from build123d import *

# Parameters (mm, degrees)
SKETCH1_W           = 55
SKETCH1_H           = 35
BOSS_EXTRUDE1_DEPTH = 1.5
SKETCH2_W           = 15
SKETCH2_H           = 41
BOSS_EXTRUDE2_DEPTH = 1.5
SKETCH3_R           = 1.125
CUT_EXTRUDE1_DEPTH  = 10


with BuildPart() as part:
    # Sketch1 → Boss-Extrude1 (new body)
    with BuildSketch(Plane(origin=(0, 0, 0), x_dir=(1, 0, 0), z_dir=(0, 1, 0))):
        Rectangle(SKETCH1_W, SKETCH1_H)
    extrude(amount=BOSS_EXTRUDE1_DEPTH)

    # Sketch2 → Boss-Extrude2 (add)
    with BuildSketch(Plane(origin=(0, 0, 0), x_dir=(1, 0, 0), z_dir=(0, 1, 0))):
        with Locations((35, 0)):
            Rectangle(SKETCH2_W, SKETCH2_H)
        with Locations((-35, 0)):
            Rectangle(SKETCH2_W, SKETCH2_H)
    extrude(amount=BOSS_EXTRUDE2_DEPTH)

    # Sketch3 → Cut-Extrude1 (cut)
    with BuildSketch(Plane(origin=(0, 0, 0), x_dir=(1, 0, 0), z_dir=(0, 1, 0))):
        with Locations(Location((-39.5, -16.5, 0), (0, 0, 270))):
            Circle(SKETCH3_R)
        with Locations(Location((-39, -7.5, 0), (0, 0, 270))):
            Circle(SKETCH3_R)
        with Locations(Location((-39, 7.5, 0), (0, 0, 270))):
            Circle(SKETCH3_R)
        with Locations(Location((-39.5, 16.5, 0), (0, 0, 270))):
            Circle(SKETCH3_R)
        with Locations(Location((-18, 15, 0), (0, 0, 270))):
            Circle(SKETCH3_R)
        with Locations(Location((18, 15, 0), (0, 0, 270))):
            Circle(SKETCH3_R)
        with Locations(Location((-18, -15, 0), (0, 0, 270))):
            Circle(SKETCH3_R)
        with Locations(Location((18, -15, 0), (0, 0, 270))):
            Circle(SKETCH3_R)
    cut_extrude1 = extrude(amount=CUT_EXTRUDE1_DEPTH, mode=Mode.SUBTRACT)

    # Mirror1: Cut-Extrude1 across plane
    add(cut_extrude1.mirror(Plane(origin=(0, 0, 0), x_dir=(0, 0, 1), z_dir=(1, 0, 0))), mode=Mode.SUBTRACT)


solid = part.part
Design review of the part built by this model. Coordinates are the model's own, in mm. A direction names the side the tool comes from. Coordinates: 2 decimals unless noted, no trailing zeros. Write each loop counter-clockwise with the first axis right and the second up, starting at its lowest first coordinate (ties: lowest second). Pieces come first, ordered by that corner, then holes. Notation, with made-up numbers: (-2, 37.5) - (19, 37.5) arc R12 ccw to (19, 50.5) - close; hole circle Ø4 at (85.25, 85.5). An arc over 180 degrees is marked (long way). One line per item, written item: value.
1) To check wall thickness, follow probe 1 along X at (y, z) = (0.6, 15) (3 decimals); probe 2 along X at (y, z) = (0.95, -7.5) (3 decimals); probe 3 along Z at (x, y) = (39, 1) (3 decimals). State the ranges of each line that lie inside material, in increasing order.
Answer sheet:
probe 1: x = -42.5 to -19.125, -16.875 to 16.875, 19.125 to 42.5
probe 2: x = -42.5 to -40.125, -37.875 to 37.875, 40.125 to 42.5
probe 3: z = -20.5 to -17.508, -15.492 to -8.625, -6.375 to 6.375, 8.625 to 15.492, 17.508 to 20.5
2) Add section D-D (x = -14.5). State the section outline as (y, z) points, plus the area to 3 significant figures.
Answer sheet:
outline: (0, -17.5) - (1.5, -17.5) - (1.5, 17.5) - (0, 17.5) - close
area: 52.5 mm2
3) Insertion check: pin 1 (2 mm diameter, centred on x = -39.5, z = -16.5, fed in from -Y). The pin has a flat end and moves straight along its axis. Give the tip position at first contact, or say it passes through.
Answer sheet:
pin 1: passes through
4) Add section B-B (z = 7.5). State the section outline as (x, y) points (3 decimals).
Answer sheet:
outline: (-42.5, 0) - (-40.125, 0) - (-40.125, 1.5) - (-42.5, 1.5) - close; (-37.875, 0) - (37.875, 0) - (37.875, 1.5) - (-37.875, 1.5) - close; (40.125, 0) - (42.5, 0) - (42.5, 1.5) - (40.125, 1.5) - close
5) Mouldability with a two-part tool opening along Z and no side actions: class faces 1 (the face through (-40.6, 0.74, -16.74)), 2 (the face through (42.5, 1, 0)), 3 (the face through (-35, 1, -20.5)) as +Z half, -Z half, draft (parallel to the pull), parting line (faces both ways), or undercut.
Answer sheet:
face 1: undercut
face 2: draft
face 3: -Z half
6) Add section C-C (y = 1.15). Give the number of separate pieces and of enclosed holes in the cut face, plus the area to 3 significant figures.
Answer sheet:
separate pieces: 1
enclosed holes: 12
area: 3,110 mm2
7) For faces 4 (the face through (0, 1, -17.5)), 5 (the face through (-17.05, 0.74, -14.4)), 6 (the face through (-27.5, 1, 19)), list the 3-axis set-ups (+Z, -Z, +X, -X, +Y, -Y) from which the entire face can be reached by the end or side of a thin tool; tool diameter is ignored.
Answer sheet:
face 4: -Z, +Y, -Y
face 5: +Y, -Y
face 6: +Z, +Y, -Y
8) Add section A-A (x = 18). State the section outline as (y, z) points (3 decimals), plus the area to 4 significant figures.
Answer sheet:
outline: (0, -17.5) - (1.5, -17.5) - (1.5, -16.125) - (0, -16.125) - close; (0, -13.875) - (1.5, -13.875) - (1.5, 13.875) - (0, 13.875) - close; (0, 16.125) - (1.5, 16.125) - (1.5, 17.5) - (0, 17.5) - close
area: 45.75 mm2
